```python
from build123d import *

# Parameters (mm, degrees)
F0_W             = 53.254
F0_H             = 20
F0_H_2           = 31.75
F1_DEPTH         = 45
F2_W             = 53.254
F2_H             = 20
F3_DEPTH         = 15
F4_R             = 31.1332376333
F5_DEPTH         = 20
F6_R             = 31.1332376333
F7_DEPTH         = 20
F8_R             = 17.5
F9_DEPTH         = 100
F11_DEPTH        = 100
F11_COPIES_COUNT = 8


# Not quite as in the source:
# - a pattern or mirror of a feature is missing from the dataset's text; its kind, count and spacing are read off the source's solid


with BuildPart() as f1:
    # F0 (on Top) → F1 (new body)
    with BuildSketch(Plane.XY):
        with Locations((0, 25.875)):
            Rectangle(F0_W, F0_H)
        Rectangle(F0_W, F0_H_2)
        with Locations((0, -25.875)):
            Rectangle(F0_W, F0_H)
    extrude(amount=F1_DEPTH)

    # F2 (on face) → F3 (join)
    with BuildSketch(Plane.XY.offset(45)):
        with Locations((0, 25.875)):
            Rectangle(F2_W, F2_H)
        with Locations((0, -25.875)):
            Rectangle(F2_W, F2_H)
    extrude(amount=F3_DEPTH)

    # F4 (on face) → F5 (join)
    with BuildSketch(Plane.XZ.offset(-15.875)):
        with Locations((0, 76.1332376333)):
            Circle(F4_R)
    extrude(amount=-F5_DEPTH)

    # F6 (on face) → F7 (join)
    with BuildSketch(Plane(origin=(0, -15.875, 0), x_dir=(-1, 0, 0), z_dir=(0, 1, 0))):
        with Locations((0, 76.1332376333)):
            Circle(F6_R)
    extrude(amount=-F7_DEPTH)

    # F8 (on face) → F9 (cut)
    with BuildSketch(Plane(origin=(0, 35.875, 0), x_dir=(-1, 0, 0), z_dir=(0, 1, 0))):
        with Locations((0, 76.1332376333)):
            Circle(F8_R)
    extrude(amount=-F9_DEPTH, mode=Mode.SUBTRACT)

    # F10 (on face) → F11 (cut)
    with BuildSketch(Plane(origin=(0, 35.875, 0), x_dir=(-1, 0, 0), z_dir=(0, 1, 0))):
        with BuildLine():
            ThreePointArc((0, 102.19985645), (-1.75, 100.44985645), (0, 98.69985645))
            Line((0, 98.69985645), (0, 102.19985645))
        make_face()
        with BuildLine():
            Line((0, 102.19985645), (0, 98.69985645))
            ThreePointArc((0, 98.69985645), (1.2374368671, 99.2124195829), (1.75, 100.44985645))
            ThreePointArc((1.75, 100.44985645), (1.2374368671, 101.6872933171), (0, 102.19985645))
        make_face()
    f11 = extrude(amount=-F11_DEPTH, mode=Mode.SUBTRACT)

    # F11_copies: F11 ×8 about axis
    f11_copies_axis = Axis((0, 0, 76.133238), (0, 1, 0))
    for i in range(1, F11_COPIES_COUNT):
        add(f11.rotate(f11_copies_axis, i * 360 / F11_COPIES_COUNT), mode=Mode.SUBTRACT)


solid = f1.part
```
For this review, take the finished solid that the model builds, in its own axes (mm). A direction names the side the tool comes from. Coordinates: 2 decimals unless noted, no trailing zeros. Write each loop counter-clockwise with the first axis right and the second up, starting at its lowest first coordinate (ties: lowest second). Pieces come first, ordered by that corner, then holes. Notation, with made-up numbers: (56.25, 41.5) -> (92.25, 41.5) arc R31 ccw to (92.25, 68.5) -> close; hole circle Ø2 at (-22.75, 63). An arc over 180 degrees is marked (long way). Put each result on its own line as item: value.
Q1. Tool access review of faces 5 (the flat face through (0, 1, 0)), 6 (the flat face through (-26.627, -1, 30)), 7 (the flat face through (0, 0, 45)), 8 (the flat face through (26.627, -1, 30)): name each direction out of +Z, -Z, +X, -X, +Y, -Y from which nothing blocks a thin tool from reaching the whole face with its end or side.
From the geometry:
face 5: -Z, +X, -X, +Y, -Y
face 6: -Z, -X, +Y, -Y
face 7: +Z, +X, -X
face 8: -Z, +X, +Y, -Y
Q2. Wall thickness on L1, parallel to Y at x = -26.5, z = 64 (3 decimals); L2, parallel to Z at x = -16, y = 30; L3, parallel to Z at x = 14, y = -25: over which ranges is each line inside the solid? List them lowest first.
From the geometry:
L1: y = -35.875 to -15.875, 15.875 to 35.875
L2: z = 0 to 57.66, 60.22 to 69.04, 83.22 to 92.05, 94.61 to 102.84
L3: z = 0 to 65.63, 86.63 to 103.94
Q3. Take a section at A-A, the plane y = -20. Count the separate pieces of the cut face and the enclosed holes in it, then the cut area to 3 significant figures.
From the geometry:
separate pieces: 1
enclosed holes: 9
area: 4,640 mm2
Q4. Take a section at C-C, the plane z = 96.5. State the section outline as (x, y) points (3 decimals).
From the geometry:
outline: (-23.547, -35.875) -> (23.547, -35.875) -> (23.547, -15.875) -> (-23.547, -15.875) -> close; (-23.547, 15.875) -> (23.547, 15.875) -> (23.547, 35.875) -> (-23.547, 35.875) -> close
Q5. The part is to be moulded in two halves that separate along Y. For faces 1 (the cylindrical face through (0.922, 25.735, 107.253)), 2 (the flat face through (-13, -15.875, 63)), 3 (the flat face through (0, 35.875, 42)), 4 (the flat face through (0, -35.875, 42)), say which applies: +Y half, -Y half, draft (parallel to the pull), parting line (faces both ways), or undercut.
From the geometry:
face 1: draft
face 2: undercut
face 3: +Y half
face 4: -Y half
Q6. Take a section at B-B, the plane z = 84.5. State the section outline as (x, y) points (3 decimals).
From the geometry:
outline: (-29.988, -35.875) -> (-15.37, -35.875) -> (-15.37, -15.875) -> (-29.988, -15.875) -> close; (-29.988, 15.875) -> (-15.37, 15.875) -> (-15.37, 35.875) -> (-29.988, 35.875) -> close; (15.37, -35.875) -> (29.988, -35.875) -> (29.988, -15.875) -> (15.37, -15.875) -> close; (15.37, 15.875) -> (29.988, 15.875) -> (29.988, 35.875) -> (15.37, 35.875) -> close
Q7. Take a section at D-D, the plane x = 10. State the section outline as (y, z) points (3 decimals).
From the geometry:
outline: (-35.875, 0) -> (35.875, 0) -> (35.875, 61.772) -> (15.875, 61.772) -> (15.875, 45) -> (-15.875, 45) -> (-15.875, 61.772) -> (-35.875, 61.772) -> close; (-35.875, 90.495) -> (-15.875, 90.495) -> (-15.875, 105.617) -> (-35.875, 105.617) -> close; (15.875, 90.495) -> (35.875, 90.495) -> (35.875, 105.617) -> (15.875, 105.617) -> close
Q8. Clearance check with flat-ended pins moving along their axes: pin 1 Ø4 at (x, y) = (15.5, 5) entering from -Z; pin 2 Ø4 at (y, z) = (16.5, 67) entering from -X; pin 3 Ø1 at (y, z) = (1, 15) entering from -X; pin 4 Ø16 at (x, y) = (9.5, -1) entering from +Z. State where each tip first meets the part, or that it passes through.
From the geometry:
pin 1: stops at z = 0
pin 2: stops at x = -30.31
pin 3: stops at x = -26.63
pin 4: stops at z = 45
